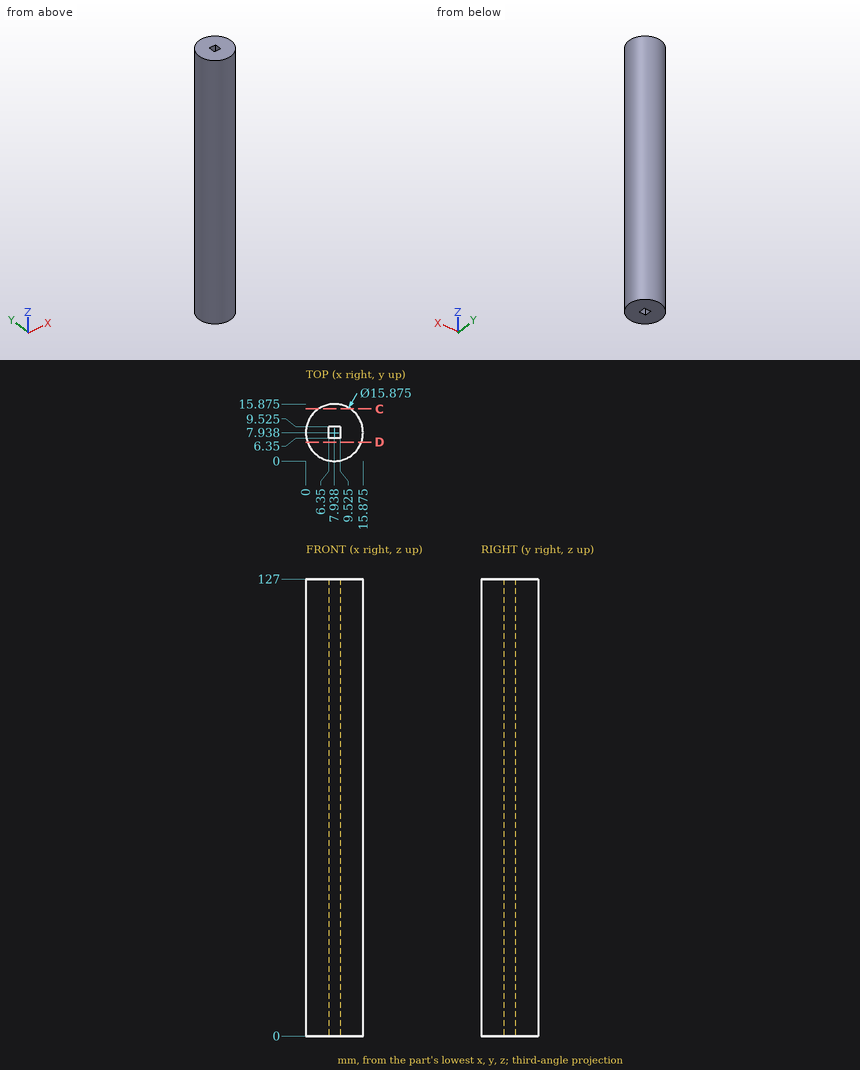
For this review, use the dimensioned drawing (mm, ordinates from the lowest corner) and the shaded views. Give positions to 0.01 mm unless a question says otherwise; leave off trailing zeros. Write each loop counter-clockwise with the first axis right and the second up, starting at its lowest first coordinate (ties: lowest second). Pieces come first, ordered by that corner, then holes. Notation, with made-up numbers: M 70,31.25 L 113,31.25 A29 ccw 113,65.25 Z; hole C 75.25,-8.5 d6. An arc over 180 degrees is marked long. Answer as a JSON object with one key per item and string values. Group by question number.
Item 1: Consider section C-C on y = 14.5. Write out the cut boundary in (x, z).
Item 2: For probe 1 along X at (y, z) = (2.5, 75) (1 decimal); probe 2 along X at (y, z) = (14.75, 86.5) (1 decimal); probe 3 along Y at (x, z) = (9.75, 99) (1 decimal), list the stretches that pass through material, from the lowest coordinate up. Write a range as [from, to].
Item 3: Consider section D-D on y = 5.25. Write out the cut boundary in (x, z), plus the area to 3 significant figures.
Item 4: For pin 1 Ø2 at (y, z) = (3, 101.5) entering from +X; pin 2 Ø4 at (x, z) = (12.5, 59) entering from +Y; pin 3 Ø1 at (y, z) = (4, 93.5) entering from +X, all flat-tipped, find the tip position at first contact; note any pin that passes through.
Check result:
{
 "1": {"outline": "M 3.47,0 L 12.4,0 L 12.4,127 L 3.47,127 Z"},
 "2": {"probe 1": "x = [2.2, 13.7]", "probe 2": "x = [3.9, 12]", "probe 3": "y = [0.2, 15.7]"},
 "3": {"outline": "M 0.47,0 L 15.41,0 L 15.41,127 L 0.47,127 Z", "area": "1,900 mm^2"},
 "4": {"pin 1": "stops at x = 14.83", "pin 2": "stops at y = 15.45", "pin 3": "stops at x = 15.09"}
}
